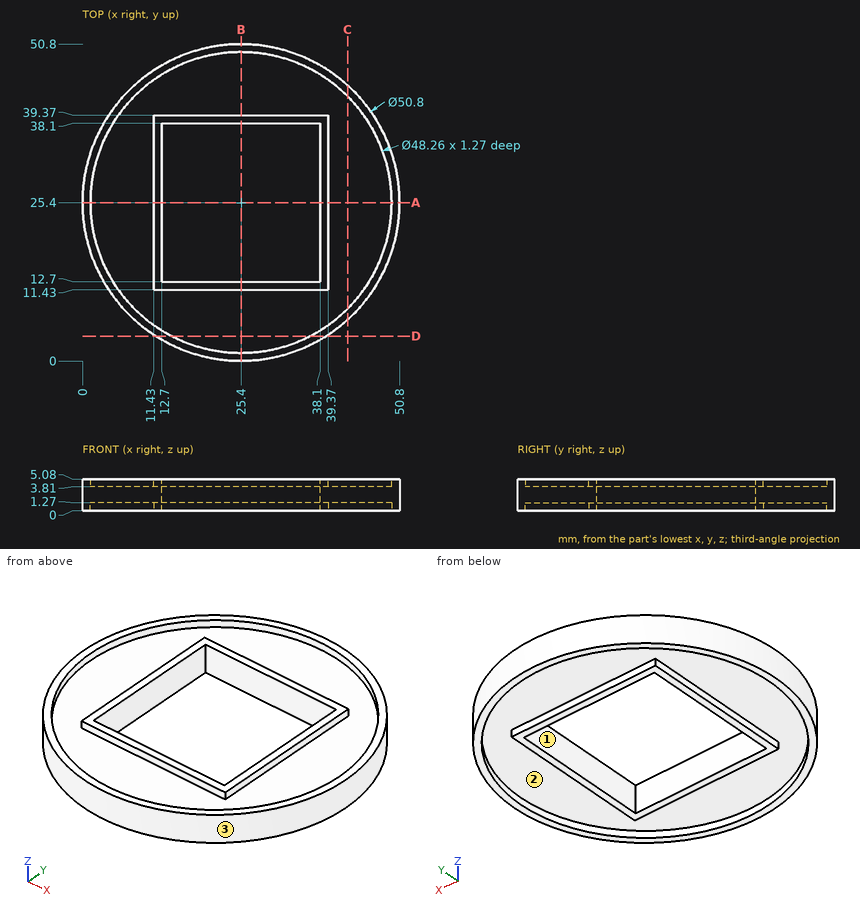
Verification items for this drawing (mm, ordinates from the low corner). Coordinates: 2 decimals unless noted, no trailing zeros. Order: outer loops, then holes, each group sorted by start corner. A loop starts at its lowest first (then second) coordinate and runs counter-clockwise, first axis right, second up. Notation, with made-up numbers: (-31, 11.5) - (-21, 11.5) arc R11 cw to (-21, 15.5) - close; hole circle Ø7 at (-10, 6). An arc over 180 degrees is marked (long way). Use one line per item in the form item = value.
1. Section check D-D (y = 4). Record the boundary of the cut face in (x, z).
Here are the results:
outline = (11.72, 0) - (14.25, 0) - (14.25, 1.27) - (36.55, 1.27) - (36.55, 0) - (39.08, 0) - (39.08, 5.08) - (36.55, 5.08) - (36.55, 3.81) - (14.25, 3.81) - (14.25, 5.08) - (11.72, 5.08) - close
2. Gauge pin test, flat ends, axial feed: pin 1 (1 mm diameter, centred on y = 31.5, z = 0.5, fed in from +X) (3 decimals); pin 2 (2.5 mm diameter, centred on y = 20.5, z = 3.5, fed in from +X); pin 3 (1 mm diameter, centred on y = 18.5, z = 1, fed in from -X). Record the tip position at first contact, or that the pin passes through.
Here are the results:
pin_1 = 50.175
pin_2 = 50.54
pin_3 = 0.82
3. Section check C-C (x = 42.5). Record the boundary of the cut face in (y, z).
Here are the results:
outline = (6.62, 0) - (8.38, 0) - (8.38, 1.27) - (42.42, 1.27) - (42.42, 0) - (44.18, 0) - (44.18, 5.08) - (42.42, 5.08) - (42.42, 3.81) - (8.38, 3.81) - (8.38, 5.08) - (6.62, 5.08) - close
4. Section check A-A (y = 25.4). Record the boundary of the cut face in (x, z), then the cut area to 3 significant figures.
Here are the results:
outline = (0, 0) - (1.27, 0) - (1.27, 1.27) - (11.43, 1.27) - (11.43, 0) - (12.7, 0) - (12.7, 5.08) - (11.43, 5.08) - (11.43, 3.81) - (1.27, 3.81) - (1.27, 5.08) - (0, 5.08) - close; (38.1, 0) - (39.37, 0) - (39.37, 1.27) - (49.53, 1.27) - (49.53, 0) - (50.8, 0) - (50.8, 5.08) - (49.53, 5.08) - (49.53, 3.81) - (39.37, 3.81) - (39.37, 5.08) - (38.1, 5.08) - close
area = 77.4 mm²
5. Draft check along Y on the marked faces 1, 2 and 3. Enter one of: pulls with the +Y half, pulls with the -Y half, needs draft (parallel to the pull), parting line crosses it, or undercut.
Here are the results:
face_1 = undercut
face_2 = undercut
face_3 = parting line crosses it
6. Scan lines: line 1 (Y direction, x = 25.4, z = 4.45); line 2 (Y direction, x = 25, z = 1.7). Record each from-to range of solid material in increasing order.
Here are the results:
line_1 = 0 to 1.27, 11.43 to 12.7, 38.1 to 39.37, 49.53 to 50.8
line_2 = 0 to 12.7, 38.1 to 50.8
